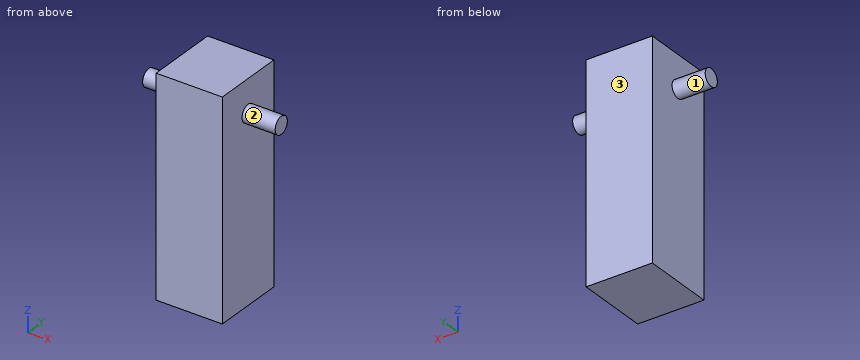
from build123d import *

# Parameters (mm, degrees)
CROQUIS1_W              = 20
CROQUIS1_H              = 65
SALIENTE_EXTRUIR1_DEPTH = 11
CROQUIS3_R              = 2.6
SALIENTE_EXTRUIR2_DEPTH = 20


with BuildPart() as part:
    # Croquis1 → Saliente-Extruir1 (new, symmetric)
    with BuildSketch(Plane(origin=(0, 0, 0), x_dir=(1, 0, 0), z_dir=(0, 1, 0))):
        Rectangle(CROQUIS1_W, CROQUIS1_H)
    extrude(amount=SALIENTE_EXTRUIR1_DEPTH, both=True)

    # Croquis3 → Saliente-Extruir2 (add, symmetric)
    with BuildSketch(Plane.ZY):
        with Locations(Location((22.5, 0, 0), (0, 0, 180))):
            Circle(CROQUIS3_R)
    extrude(amount=SALIENTE_EXTRUIR2_DEPTH, both=True)


solid = part.part
Source: CAD feature listing. Evaluate the final solid. Frame: model axes, mm. Face numbers are marked on the shaded views. A direction names the side the tool comes from. Round coordinates to 2 decimals unless told otherwise and drop trailing zeros. Loops run counter-clockwise (first coordinate to the right, second up) from the corner with the lowest first, then second, coordinate; pieces in that order, holes last.
Q1. Section A-A, the plane y = 0. Return loops of the section in (x, z).
Q2. Ray query, line 1 (X direction, y = -9.5, z = -12); line 2 (Z direction, x = -10.5, y = -1.25); line 3 (Y direction, x = -14, z = 22). Return the intervals inside material, ascending.
Q3. Section B-B, the plane z = 22.5. Return loops of the section in (x, y).
Q4. First-contact query: P1, Ø2, axis at y = 8.5, z = 17, coming from the +X side; P2, Ø6.5, axis at y = -5, z = -15.5, coming from the -X side; P3, Ø1.5, axis at x = -13.5, y = 3.5, coming from the -Z side. Flat tips, straight axial feed; report the tip coordinate or a pass-through.
Q5. Access query for the marked faces 1, 2 and 3. Directions: +Z, -Z, +X, -X, +Y, -Y. A direction counts if a zero-diameter tool reaches every point of the face in a straight line with its end or side. Return the directions, or none.
Q6. Section C-C, the plane x = -15. Return loops of the section in (y, z), plus the area to 3 significant figures.
Q7. Section D-D, the plane z = -27. Return loops of the section in (x, y).
Solutions:
1. outline: (-20, 19.9) - (-10, 19.9) - (-10, -32.5) - (10, -32.5) - (10, 19.9) - (20, 19.9) - (20, 25.1) - (10, 25.1) - (10, 32.5) - (-10, 32.5) - (-10, 25.1) - (-20, 25.1) - close
2. line 1: x = -10 to 10
2. line 2: z = 20.22 to 24.78
2. line 3: y = -2.55 to 2.55
3. outline: (-20, -2.6) - (-10, -2.6) - (-10, -11) - (10, -11) - (10, -2.6) - (20, -2.6) - (20, 2.6) - (10, 2.6) - (10, 11) - (-10, 11) - (-10, 2.6) - (-20, 2.6) - close
4. P1: stops at x = 10
4. P2: stops at x = -10
4. P3: passes through
5. face 1: -X
5. face 2: +X
5. face 3: +Z, -Z, +X, -X, +Y
6. outline: circle Ø5.2 at (0, 22.5)
6. area: 21.2 mm2
7. outline: (-10, -11) - (10, -11) - (10, 11) - (-10, 11) - close
